CAD build for the part. Positions are in the model's coordinates, mm. A direction names the side the tool comes from. Round coordinates to 2 decimals unless told otherwise and drop trailing zeros. Loops run counter-clockwise (first coordinate to the right, second up) from the corner with the lowest first, then second, coordinate; pieces in that order, holes last. Notation, with made-up numbers: M 13,35 L 41,35 A14 cw 41,43 Z; hole C 30,59 d3. An arc over 180 degrees is marked long. Use a Markdown table: item, result. Add a question column.
(1) Flat gauge pins, fed straight in: P1, Ø3, axis at x = 31, z = -24, coming from the -Y side; P2, Ø5, axis at x = 12.5, z = -15.5, coming from the +Y side; P3, Ø3, axis at x = 22.5, z = -14, coming from the -Y side. Where does each tip first touch, or does it go through?
(2) Band-saw the part on D-D, the plane x = 24. Write the cut outline in (y, z).
(3) Two-plate mould, pull along X, no slides. Class faces 1 (the face through (40, 23, -14)), 2 (the face through (5.6, 42.1, -14.2)), 3 (the face through (7, 46.1, -20)), 4 (the face through (0, 23, -14)): released by +X, released by -X, zero draft, split by the parting line, or undercut.
(4) Band-saw the part on C-C, the plane z = -14. Write the cut outline in (x, y), and give its area (3 significant figures).
(5) Band-saw the part on A-A, the plane x = 17.5. Write the cut outline in (y, z), and give its area (3 significant figures).
(6) Wall check: L1, parallel to X at y = 0.8, z = -14; L2, parallel to Y at x = 34.5, z = -20.5; L3, parallel to Z at x = 17, y = 44. Give the ranges that are in metal, low to high.
(7) Which spindle directions (+Z, -Z, +X, -X, +Y, -Y) get a long thin tool onto all of the face, cutting with end or side? Do faces 5 (the face through (20.95, 44.07, -3.03)), 6 (the face through (37, 23, -28)), 7 (the face through (35, 23, -14)). Say none if no direction does.
(8) Band-saw the part on B-B, the plane y = 40. Write the cut outline in (x, z), and give its area (3 significant figures).
from build123d import *

# Parameters (mm, degrees)
SKETCH1_W           = 35
SKETCH1_H           = 28
SKETCH1_R           = 2.65
BOSS_EXTRUDE1_DEPTH = 4
SKETCH2_W           = 5
SKETCH2_H           = 28
BOSS_EXTRUDE2_DEPTH = 42.1
SKETCH3_W           = 45
SKETCH3_H           = 28
SKETCH3_R           = 11.5
BOSS_EXTRUDE3_DEPTH = 4


with BuildPart() as part:
    # Sketch1 → Boss-Extrude1 (new body)
    with BuildSketch(Plane(origin=(0, 0, 0), x_dir=(1, 0, 0), z_dir=(0, 1, 0))):
        with Locations((17.5, 14)):
            Rectangle(SKETCH1_W, SKETCH1_H)
        with Locations(Location((12.5, 14, 0), (0, 0, 270))):
            Circle(SKETCH1_R, mode=Mode.SUBTRACT)
        with Locations(Location((22.5, 14, 0), (0, 0, 270))):
            Circle(SKETCH1_R, mode=Mode.SUBTRACT)
    extrude(amount=BOSS_EXTRUDE1_DEPTH)

    # Sketch2 → Boss-Extrude2 (add)
    with BuildSketch(Plane.XZ):
        with Locations((-2.5, -14)):
            Rectangle(SKETCH2_W, SKETCH2_H)
        with Locations((37.5, -14)):
            Rectangle(SKETCH2_W, SKETCH2_H)
    extrude(amount=-BOSS_EXTRUDE2_DEPTH)

    # Sketch3 → Boss-Extrude3 (add)
    with BuildSketch(Plane(origin=(0, 42.1, 0), x_dir=(1, 0, 0), z_dir=(0, 1, 0))):
        with Locations((17.5, 14)):
            Rectangle(SKETCH3_W, SKETCH3_H)
        with Locations(Location((17.5, 14, 0), (0, 0, 270))):
            Circle(SKETCH3_R, mode=Mode.SUBTRACT)
    extrude(amount=BOSS_EXTRUDE3_DEPTH)


solid = part.part
Return value:
| question | item | result |
|---|---|---|
| 1 | P1 | y = 0 |
| 1 | P2 | y = 4 |
| 1 | P3 | through |
| 2 | outline | M 0,-28 L 4,-28 L 4,-16.18 L 0,-16.18 Z; M 0,-11.82 L 4,-11.82 L 4,0 L 0,0 Z; M 42.1,-28 L 46.1,-28 L 46.1,-23.49 L 42.1,-23.49 Z; M 42.1,-4.51 L 46.1,-4.51 L 46.1,0 L 42.1,0 Z |
| 3 | face 1 | released by +X |
| 3 | face 2 | undercut |
| 3 | face 3 | zero draft |
| 3 | face 4 | undercut |
| 4 | outline | M -5,0 L 9.85,0 L 9.85,4 L 0,4 L 0,42.1 L 6,42.1 L 6,46.1 L -5,46.1 Z; M 15.15,0 L 19.85,0 L 19.85,4 L 15.15,4 Z; M 25.15,0 L 40,0 L 40,46.1 L 29,46.1 L 29,42.1 L 35,42.1 L 35,4 L 25.15,4 Z |
| 4 | area | 607 mm^2 |
| 5 | outline | M 0,-28 L 4,-28 L 4,0 L 0,0 Z; M 42.1,-28 L 46.1,-28 L 46.1,-25.5 L 42.1,-25.5 Z; M 42.1,-2.5 L 46.1,-2.5 L 46.1,0 L 42.1,0 Z |
| 5 | area | 132 mm^2 |
| 6 | L1 | -5 to 9.85, 15.15 to 19.85, 25.15 to 40 |
| 6 | L2 | 0 to 4, 42.1 to 46.1 |
| 6 | L3 | -28 to -25.49, -2.51 to 0 |
| 7 | face 5 | +Y |
| 7 | face 6 | -Z, +X, -X, +Y, -Y |
| 7 | face 7 | +Z, -Z |
| 8 | outline | M -5,-28 L 0,-28 L 0,0 L -5,0 Z; M 35,-28 L 40,-28 L 40,0 L 35,0 Z |
| 8 | area | 280 mm^2 |
